Part print with two shaded views. Sizes in mm from the minimum x, y, z corner. A direction names the side the tool comes from. Give positions to 0.01 mm unless a question says otherwise; leave off trailing zeros. Write each loop counter-clockwise with the first axis right and the second up, starting at its lowest first coordinate (ties: lowest second). Pieces come first, ordered by that corner, then holes. Notation, with made-up numbers: (56, -6.5) - (104, -6.5) arc R29 cw to (104, 16.5) - close; hole circle Ø1 at (17, 43.25). An arc over 180 degrees is marked (long way). Answer as a JSON object with one key per item and string values.
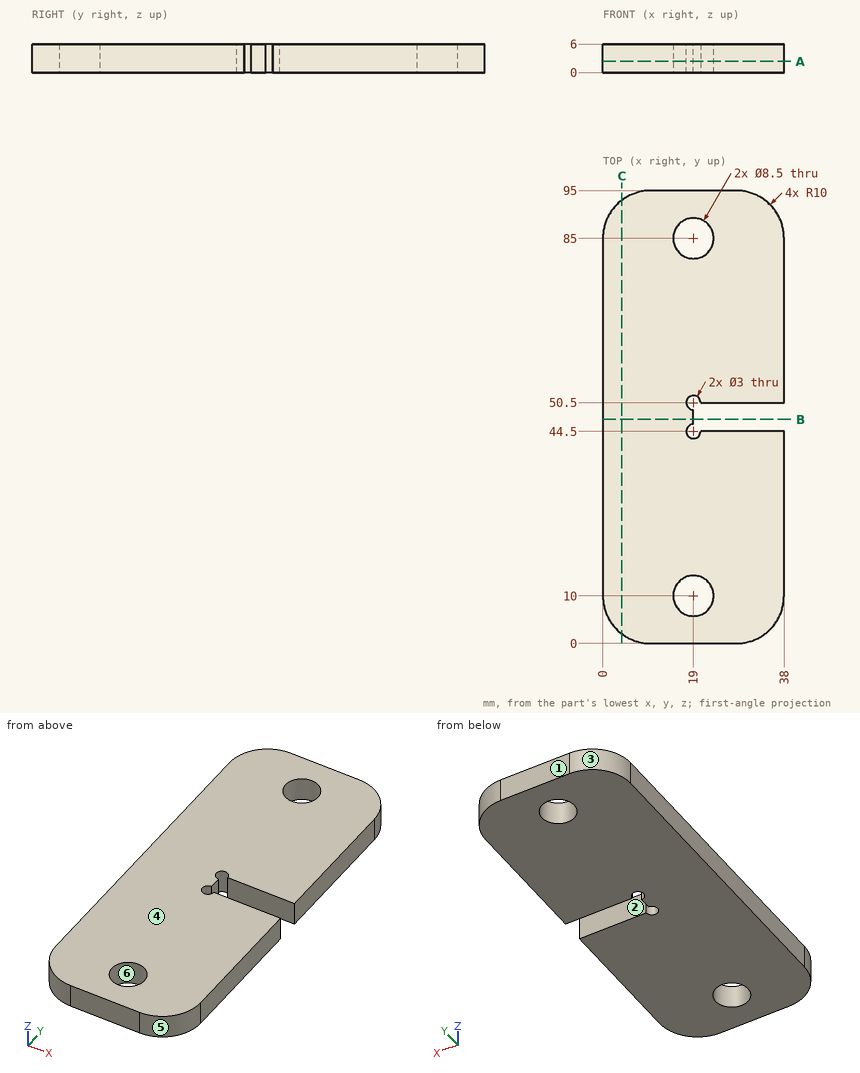
(1) Pull direction X, two halves, no side cores. Call the marked faces 3, 4, 5 and 6: pulls with the +X half, pulls with the -X half, needs draft (parallel to the pull), parting line crosses it, or undercut.
Answer key:
{"face 3": "pulls with the -X half", "face 4": "needs draft", "face 5": "pulls with the +X half", "face 6": "undercut"}
(2) Saw through at C-C, the plane x = 4. Give the cut face in (y, z).
Answer key:
{"outline": "(2, 0) - (93, 0) - (93, 6) - (2, 6) - close"}
(3) Saw through at A-A, the plane z = 2.35. Give the cut face in (x, y), and give its area (3 significant figures).
Answer key:
{"outline": "(0, 10) arc R10 ccw to (10, 0) - (28, 0) arc R10 ccw to (38, 10) - (38, 44.5) - (20.5, 44.5) arc R1.5 cw (long way) to (19, 46) - (19, 49) arc R1.5 cw (long way) to (20.5, 50.5) - (38, 50.5) - (38, 85) arc R10 ccw to (28, 95) - (10, 95) arc R10 ccw to (0, 85) - close; hole circle Ø8.5 at (19, 10); hole circle Ø8.5 at (19, 85)", "area": "3,290 mm²"}
(4) Saw through at B-B, the plane y = 47. Give the cut face in (x, z).
Answer key:
{"outline": "(0, 0) - (19, 0) - (19, 6) - (0, 6) - close"}
(5) Probe L1, parallel to Y at x = 16.5, z = 1.3; L2, parallel to Y at x = 34.5, z = 5; L3, parallel to Y at x = 17, z = 3.25. List the from-to ranges inside material, lowest first. Write a range as [from, to].
Answer key:
{"L1": "y = [0, 6.56], [13.44, 81.56], [88.44, 95]", "L2": "y = [2.4, 44.5], [50.5, 92.6]", "L3": "y = [0, 6.25], [13.75, 81.25], [88.75, 95]"}
(6) 3-axis set-ups, long thin cutter, end or side, ignore diameter. For the marked faces 1 and 2: which of +Z, -Z, +X, -X, +Y, -Y reach the whole face in a straight line?
Answer key:
{"face 1": "+Z, -Z, +X, -X, +Y", "face 2": "+Z, -Z, +X"}
(7) Flat gauge pins, fed straight in: P1, Ø2.5, axis at y = 47.5, z = 2, coming from the +X side; P2, Ø3, axis at y = 43, z = 3.5, coming from the -X side. Where does each tip first touch, or does it go through?
Answer key:
{"P1": "stops at x = 19", "P2": "stops at x = 0"}
